from build123d import *

# Parameters (mm, degrees)
BOSS_EXTRUDE1_DEPTH      = 10
FILLET1_R                = 0.3325
CIRPATTERN1_COUNT        = 15
FILLET1_OF_CIRPATTERN1_R = 0.3325
CUT_EXTRUDE1_START       = -10
CUT_EXTRUDE1_DEPTH       = 10


# Read off the part's stored shape, not the designer's step: Cut-Extrude1
with BuildPart() as part:
    # Sketch1 → Boss-Extrude1 (new body)
    with BuildSketch(Plane.XY):
        with BuildLine():
            Line((13.268609193, 0.579319988), (13.28125, 0))
            Line((13.28125, 0), (13.268609193, -0.579319988))
            ThreePointArc((13.268609193, -0.579319988), (11.2692337, -0.978550661), (9.230406341, -0.9701548))
            ThreePointArc((9.230406341, -0.9701548), (9.166982411, -1.451907379), (9.078432419, -1.92968038))
            Line((9.078432419, -1.92968038), (0, 0))
            Line((0, 0), (9.078432419, 1.92968038))
            ThreePointArc((9.078432419, 1.92968038), (9.166982411, 1.451907379), (9.230406341, 0.9701548))
            ThreePointArc((9.230406341, 0.9701548), (11.2692337, 0.978550661), (13.268609193, 0.579319988))
        make_face()
    boss_extrude1 = extrude(amount=BOSS_EXTRUDE1_DEPTH)

    # Fillet1
    fillet1_edges = [part.edges().sort_by_distance(p)[0] for p in [
        (9.230406341, 0.9701548, 5),
        (9.230406341, -0.9701548, 5),
    ]]
    fillet(fillet1_edges, radius=FILLET1_R)

    # CirPattern1: Boss-Extrude1 ×15 about axis
    cirpattern1_axis = Axis((0, 0, 0), (0, 0, 1))
    for i in range(1, CIRPATTERN1_COUNT):
        add(boss_extrude1.rotate(cirpattern1_axis, i * 360 / CIRPATTERN1_COUNT))

    # Fillet1 of CirPattern1
    fillet1_of_cirpattern1_edges = [part.edges().sort_by_distance(p)[0] for p in [
        (8.037798279, 4.640625, 5),
        (8.826993292, 2.868063979, 5),
        (5.455381873, 7.508688979, 5),
        (6.897312911, 6.21036844, 5),
        (1.92968038, 9.078432419, 5),
        (3.775024469, 8.478843779, 5),
        (-1.92968038, 9.078432419, 5),
        (0, 9.28125, 5),
        (-5.455381873, 7.508688979, 5),
        (-3.775024469, 8.478843779, 5),
        (-8.037798279, 4.640625, 5),
        (-6.897312911, 6.21036844, 5),
        (-9.230406341, 0.9701548, 5),
        (-8.826993292, 2.868063979, 5),
        (-8.826993292, -2.868063979, 5),
        (-9.230406341, -0.9701548, 5),
        (-6.897312911, -6.21036844, 5),
        (-8.037798279, -4.640625, 5),
        (-3.775024469, -8.478843779, 5),
        (-5.455381873, -7.508688979, 5),
        (0, -9.28125, 5),
        (-1.92968038, -9.078432419, 5),
        (3.775024469, -8.478843779, 5),
        (1.92968038, -9.078432419, 5),
        (6.897312911, -6.21036844, 5),
        (5.455381873, -7.508688979, 5),
        (8.826993292, -2.868063979, 5),
        (8.037798279, -4.640625, 5),
    ]]
    fillet(fillet1_of_cirpattern1_edges, radius=FILLET1_OF_CIRPATTERN1_R)

    # Cut-Extrude1 outline → Cut-Extrude1 (cut)
    with BuildSketch(Plane(origin=(0, 0, 0), x_dir=(-1, 0, 0), z_dir=(0, 0, -1)).offset(CUT_EXTRUDE1_START)):
        with BuildLine():
            Line((2.540177159, 1.5), (-2.540177159, 1.5))
            ThreePointArc((-2.540177159, 1.5), (0, -2.95), (2.540177159, 1.5))
        make_face()
    extrude(amount=CUT_EXTRUDE1_DEPTH, mode=Mode.SUBTRACT)


solid = part.part
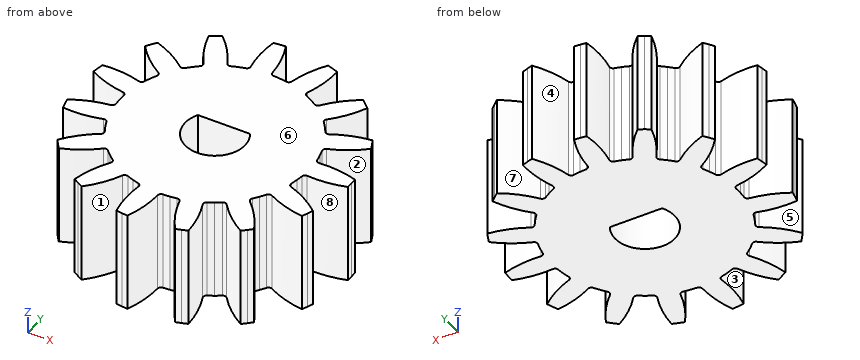
Geometry: final body of the model. Coordinates: model frame, mm. Face numbers are marked on the shaded views. A direction names the side the tool comes from. Give positions to 0.01 mm unless a question says otherwise; leave off trailing zeros. Write each loop counter-clockwise with the first axis right and the second up, starting at its lowest first coordinate (ties: lowest second). Pieces come first, ordered by that corner, then holes.
(1) Ray query, line 1 (X direction, y = 0, z = 7); line 2 (Y direction, x = 7.5, z = 5.5); line 3 (X direction, y = -9.5, z = 8). Return the intervals inside material, ascending.
(2) Mould query, pull axis Y, two halves, no side actions, for the marked faces 6, 7 and 8. Classes: released by +Y, released by -Y, zero draft, split by the parting line, or undercut.
(3) Cut plane A-A, the plane x = -10. Return loops of the section in (y, z), then the cut area to 3 significant figures.
(4) Access query for the marked faces 1, 2, 3, 4 and 5. Directions: +Z, -Z, +X, -X, +Y, -Y. A direction counts if a zero-diameter tool reaches every point of the face in a straight line with its end or side. Return the directions, or none.
(5) First-contact query: P1, Ø8, axis at x = -6, y = 0.5, coming from the -Z side; P2, Ø5, axis at y = 5, z = 5.5, coming from the +X side; P3, Ø1.5, axis at x = -7, z = 5, coming from the +Y side; P4, Ø3, axis at x = -7.5, z = 4.5, coming from the -Y side. Flat tips, straight axial feed; report the tip coordinate or a pass-through.
Values follow:
1. line 1: x = -9.28 to -2.95, 2.95 to 13.28
1. line 2: y = -9.6 to -6.8, -5.47 to 5.47, 6.8 to 9.6
1. line 3: x = -6.58 to -4.3, -2.01 to 0.01, 2.03 to 4.17, 7.37 to 9.28
2. face 6: zero draft
2. face 7: released by +Y
2. face 8: undercut
3. outline: (-8.12, 0) - (-6.12, 0) - (-6.12, 10) - (-8.12, 10) - close; (-3.17, 0) - (-1.08, 0) - (-1.08, 10) - (-3.17, 10) - close; (1.08, 0) - (3.17, 0) - (3.17, 10) - (1.08, 10) - close; (6.12, 0) - (8.12, 0) - (8.12, 10) - (6.12, 10) - close
3. area: 82.0 mm2
4. face 1: +Z, -Z, -Y
4. face 2: +Z, -Z, +X
4. face 3: +Z, -Z
4. face 4: +Z, -Z, +Y
4. face 5: +Z, -Z, -X
5. P1: stops at z = 0
5. P2: stops at x = 12.36
5. P3: stops at y = 11.72
5. P4: stops at y = -11.78
